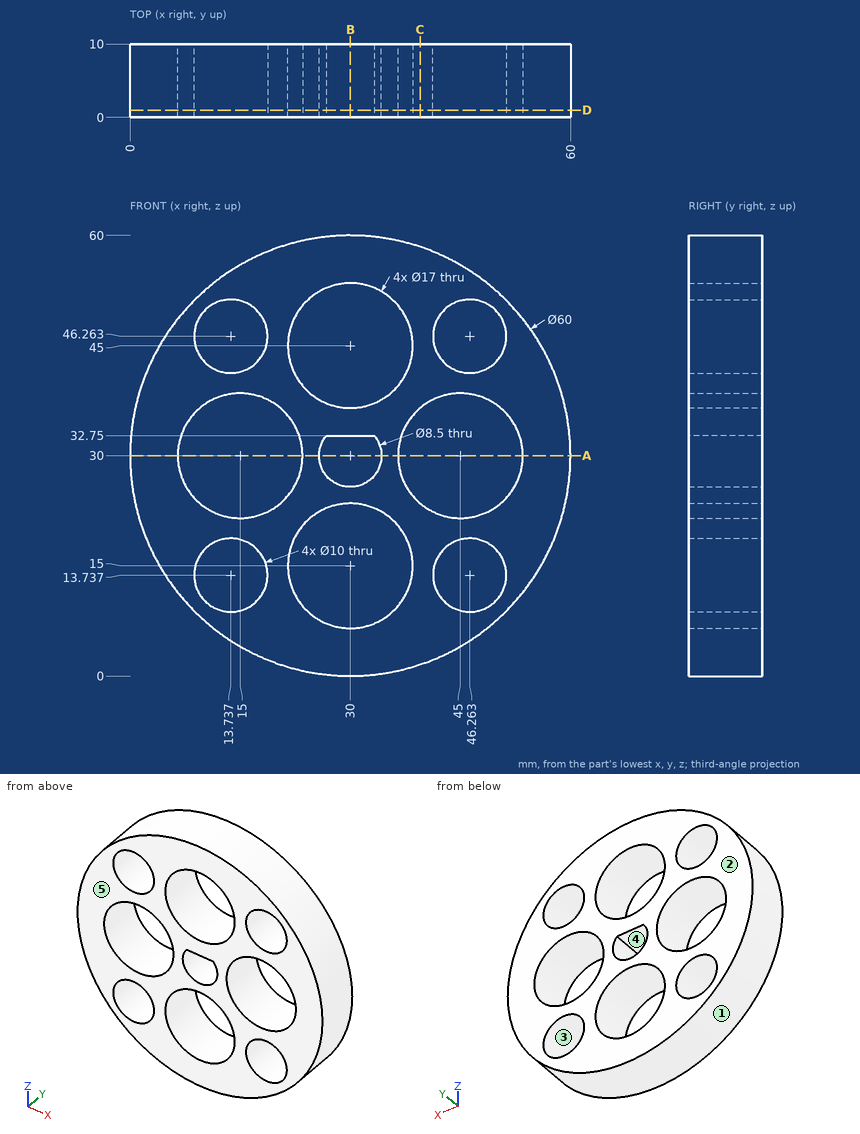
The drawing under review shows one solid part. Ordinate dimensions are in mm from its lowest x, y, z. A direction names the side the tool comes from. Coordinates: 2 decimals unless noted, no trailing zeros. Write each loop counter-clockwise with the first axis right and the second up, starting at its lowest first coordinate (ties: lowest second). Pieces come first, ordered by that corner, then holes. Notation, with made-up numbers: M -18,60.25 L 0,60.25 A29 cw 0,91.25 Z; hole C 9,62 d1. An arc over 180 degrees is marked long. Put each result on its own line as item: value.
1) Add section B-B on x = 30. Give the boundary of the cut face in (y, z).
Computed:
outline: M 0,0 L 10,0 L 10,6.5 L 0,6.5 Z; M 0,23.5 L 10,23.5 L 10,25.75 L 0,25.75 Z; M 0,32.75 L 10,32.75 L 10,36.5 L 0,36.5 Z; M 0,53.5 L 10,53.5 L 10,60 L 0,60 Z
2) For the marked faces 4 and 5, list the 3-axis set-ups (+Z, -Z, +X, -X, +Y, -Y) from which the entire face can be reached by the end or side of a thin tool; tool diameter is ignored.
Computed:
face 4: +Y, -Y
face 5: +Z, -Z, +X, -X, -Y
3) Wall thickness on probe 1 along Z at (x, y) = (30, 6.25); probe 2 along X at (y, z) = (2.75, 10) (1 decimal); probe 3 along X at (y, z) = (6, 36) (1 decimal): over which ranges is each line inside the solid? List them lowest first. Write a range as [from, to].
Computed:
probe 1: z = [0, 6.5], [23.5, 25.75], [32.75, 36.5], [53.5, 60]
probe 2: x = [7.6, 10.4], [17.1, 23.1], [36.9, 42.9], [49.6, 52.4]
probe 3: x = [0.6, 9], [21, 39], [51, 59.4]
4) Add section D-D on y = 1. State how many separate pieces and enclosed holes the cut face has.
Computed:
separate pieces: 1
enclosed holes: 9
5) Add section A-A on z = 30. Give the boundary of the cut face in (x, y).
Computed:
outline: M 0,0 L 6.5,0 L 6.5,10 L 0,10 Z; M 23.5,0 L 25.75,0 L 25.75,10 L 23.5,10 Z; M 34.25,0 L 36.5,0 L 36.5,10 L 34.25,10 Z; M 53.5,0 L 60,0 L 60,10 L 53.5,10 Z
6) Clearance check with flat-ended pins moving along their axes: pin 1 Ø1.5 at (y, z) = (4.5, 41.5) entering from +X; pin 2 Ø3 at (x, y) = (28.5, 7.5) entering from -Z; pin 3 Ø4 at (y, z) = (6, 40) entering from -X. State where each tip first meets the part, or that it passes through.
Computed:
pin 1: stops at x = 58.01
pin 2: stops at z = 0
pin 3: stops at x = 1.09
7) Add section C-C on x = 39.5. Give the boundary of the cut face in (y, z).
Computed:
outline: M 0,1.54 L 10,1.54 L 10,23.52 L 0,23.52 Z; M 0,36.48 L 10,36.48 L 10,58.46 L 0,58.46 Z
8) Draft analysis for pull direction Z (two halves, no side actions). For the marked faces 1, 2 and 3, state which applies: released by +Z, released by -Z, zero draft, split by the parting line, or undercut.
Computed:
face 1: split by the parting line
face 2: zero draft
face 3: undercut
